```python
from build123d import *

# Parameters (mm, degrees)
SKETCH2_W           = 60
SKETCH2_H           = 50
BOSS_EXTRUDE2_DEPTH = 60
SKETCH4_W           = 10
SKETCH4_H           = 20
CUT_EXTRUDE2_DEPTH  = 60
CUT_EXTRUDE4_DEPTH  = 60
SKETCH8_W           = 20
SKETCH8_H           = 20
CUT_EXTRUDE5_DEPTH  = 60
SKETCH9_W           = 20
SKETCH9_H           = 10
CUT_EXTRUDE6_DEPTH  = 40


with BuildPart() as part:
    # Sketch2 → Boss-Extrude2 (new body)
    with BuildSketch(Plane.XY):
        with Locations((2.702702703, 14.797297297)):
            Rectangle(SKETCH2_W, SKETCH2_H)
    extrude(amount=BOSS_EXTRUDE2_DEPTH)

    # Sketch4 → Cut-Extrude2 (cut)
    with BuildSketch(Plane.ZY.offset(27.297297297)):
        with Locations((5, 29.797297297)):
            Rectangle(SKETCH4_W, SKETCH4_H)
        with Locations((55, 29.797297297)):
            Rectangle(SKETCH4_W, SKETCH4_H)
    extrude(amount=-CUT_EXTRUDE2_DEPTH, mode=Mode.SUBTRACT)

    # Sketch7 → Cut-Extrude4 (cut)
    with BuildSketch(Plane(origin=(32.702702703, 0, 0), x_dir=(0, 0, -1), z_dir=(1, 0, 0))):
        Polygon((-37.5, -10.202702703), (-37.5, -0.202702703), (-45, -0.202702703), (-45, 9.797297297), (-15, 9.797297297), (-15, -0.202702703), (-22.5, -0.202702703), (-22.5, -10.202702703), align=None)
    extrude(amount=-CUT_EXTRUDE4_DEPTH, mode=Mode.SUBTRACT)

    # Sketch8 → Cut-Extrude5 (cut)
    with BuildSketch(Plane.ZY.offset(27.297297297)):
        with Locations((30, 29.797297297)):
            Rectangle(SKETCH8_W, SKETCH8_H)
    extrude(amount=-CUT_EXTRUDE5_DEPTH, mode=Mode.SUBTRACT)

    # Sketch9 → Cut-Extrude6 (cut)
    with BuildSketch(Plane.XY.offset(50)):
        with Locations((2.702702703, 34.797297297)):
            Rectangle(SKETCH9_W, SKETCH9_H)
    extrude(amount=-CUT_EXTRUDE6_DEPTH, mode=Mode.SUBTRACT)


solid = part.part
```
Check sheet for the modelled part. Datum: model origin and axes. Units: mm. A direction names the side the tool comes from. Give positions to 0.01 mm unless a question says otherwise; leave off trailing zeros. Loops run counter-clockwise (first coordinate to the right, second up) from the corner with the lowest first, then second, coordinate; pieces in that order, holes last. Notation, with made-up numbers: M 56,23.25 L 75,23.25 A17 ccw 75,45.25 Z; hole C 22,-35 d1. An arc over 180 degrees is marked long. Answer in a Markdown table with one row per item.
1) Cross-section at B-B (z = 46). Enter the section's corners in (x, y), plus the area to 3 significant figures.
Solutions:
| item | result |
|---|---|
| outline | M -27.3,-10.2 L 32.7,-10.2 L 32.7,39.8 L 12.7,39.8 L 12.7,29.8 L -7.3,29.8 L -7.3,39.8 L -27.3,39.8 Z |
| area | 2,800 mm^2 |
2) Mould release check, pull along Y, two halves, no side actions. Record for faces 5 (the face through (2, -10.203, 11)), 6 (the face through (2, 19.797, 5)), 7 (the face through (3, -0.203, 19)), 8 (the face through (2, 27, 50)): released by +Y, released by -Y, zero draft, split by the parting line, or undercut.
Solutions:
| item | result |
|---|---|
| face 5 | released by -Y |
| face 6 | released by +Y |
| face 7 | undercut |
| face 8 | zero draft |
3) Cross-section at C-C (x = -3.5). Enter the section's corners in (y, z), plus the area to 3 significant figures.
Solutions:
| item | result |
|---|---|
| outline | M -10.2,0 L 19.8,0 L 19.8,10 L 29.8,10 L 29.8,20 L 19.8,20 L 19.8,40 L 29.8,40 L 29.8,50 L 19.8,50 L 19.8,60 L -10.2,60 L -10.2,37.5 L -0.2,37.5 L -0.2,45 L 9.8,45 L 9.8,15 L -0.2,15 L -0.2,22.5 L -10.2,22.5 Z |
| area | 1,550 mm^2 |
4) Cross-section at D-D (y = -1.5). Enter the section's corners in (x, z), plus the area to 3 significant figures.
Solutions:
| item | result |
|---|---|
| outline | M -27.3,0 L 32.7,0 L 32.7,22.5 L -27.3,22.5 Z; M -27.3,37.5 L 32.7,37.5 L 32.7,60 L -27.3,60 Z |
| area | 2,700 mm^2 |
5) Cross-section at A-A (y = 22). Enter the section's corners in (x, z), plus the area to 3 significant figures.
Solutions:
| item | result |
|---|---|
| outline | M -27.3,10 L 32.7,10 L 32.7,20 L -27.3,20 Z; M -27.3,40 L 32.7,40 L 32.7,50 L -27.3,50 Z |
| area | 1,200 mm^2 |
6) Tool access check on faces 1 (the face through (3, -0.203, 41)), 2 (the face through (2, 27, 20)), 3 (the face through (12.703, 35, 15)), 4 (the face through (3, -5, 37.5)). Record the directions out of +Z, -Z, +X, -X, +Y, -Y that give a thin tool (end or side, any length) a straight path to the whole face; none if there is none.
Solutions:
| item | result |
|---|---|
| face 1 | +X, -X |
| face 2 | +X, -X, +Y |
| face 3 | +Z, -Z, +Y |
| face 4 | +X, -X, -Y |
7) Thickness scan on line 1 (Z direction, x = -6.5, y = 0); line 2 (X direction, y = 35, z = 14.5); line 3 (Y direction, x = 12, z = 42). Record the ranges inside material, lowest first.
Solutions:
| item | result |
|---|---|
| line 1 | z = 0 to 15, 45 to 60 |
| line 2 | x = -27.3 to -7.3, 12.7 to 32.7 |
| line 3 | y = -10.2 to -0.2, 9.8 to 29.8 |
8) Depth check by flat-ended pin: pin 1 (11 mm diameter, centred on x = 13.5, z = 56, fed in from +Y); pin 2 (6 mm diameter, centred on x = -2, y = 29.5, fed in from -Z); pin 3 (2 mm diameter, centred on x = 0.5, z = 29.5, fed in from -Y); pin 4 (10 mm diameter, centred on y = 26.5, z = 30, fed in from -X). Enter the tip coordinate at first touch or a pass-through.
Solutions:
| item | result |
|---|---|
| pin 1 | stops at y = 19.8 |
| pin 2 | stops at z = 10 |
| pin 3 | stops at y = 9.8 |
| pin 4 | passes through |
